from build123d import *

# Parameters (mm, degrees)
SKETCH2_W           = 94.999999992
SKETCH2_H           = 50.20499992
SKETCH2_R           = 1.5
SKETCH2_W_2         = 64.999999992
SKETCH2_H_2         = 20.20499992
BOSS_EXTRUDE2_DEPTH = 7


with BuildPart() as part:
    # Sketch2 → Boss-Extrude2 (new body)
    with BuildSketch(Plane(origin=(0, 0, 0), x_dir=(1, 0, 0), z_dir=(0, 1, 0))):
        Rectangle(SKETCH2_W, SKETCH2_H)
        with Locations(Location((-19.935762724, 17.60249996, 0), (0, 0, 270))):
            Circle(SKETCH2_R, mode=Mode.SUBTRACT)
        with Locations(Location((12.584576228, 17.60249996, 0), (0, 0, 270))):
            Circle(SKETCH2_R, mode=Mode.SUBTRACT)
        with Locations(Location((-39.970648897, 14.877942076, 0), (0, 0, 270))):
            Circle(SKETCH2_R, mode=Mode.SUBTRACT)
        with Locations(Location((-39.970648897, -2.517744737, 0), (0, 0, 270))):
            Circle(SKETCH2_R, mode=Mode.SUBTRACT)
        with Locations(Location((40.207477372, 12.990674167, 0), (0, 0, 270))):
            Circle(SKETCH2_R, mode=Mode.SUBTRACT)
        with Locations(Location((40.207477372, -3.666516508, 0), (0, 0, 270))):
            Circle(SKETCH2_R, mode=Mode.SUBTRACT)
        with Locations(Location((-13.716054438, -17.60249996, 0), (0, 0, 270))):
            Circle(SKETCH2_R, mode=Mode.SUBTRACT)
        with Locations(Location((6.580630125, -17.60249996, 0), (0, 0, 270))):
            Circle(SKETCH2_R, mode=Mode.SUBTRACT)
        Rectangle(SKETCH2_W_2, SKETCH2_H_2, mode=Mode.SUBTRACT)
    extrude(amount=BOSS_EXTRUDE2_DEPTH)


solid = part.part
Work out the finished part from the listing and answer in its coordinate system (mm). A direction names the side the tool comes from. Round coordinates to 2 decimals unless told otherwise and drop trailing zeros. Write each loop counter-clockwise with the first axis right and the second up, starting at its lowest first coordinate (ties: lowest second). Pieces come first, ordered by that corner, then holes. Notation, with made-up numbers: (49, 35) - (70, 35) arc R23 ccw to (70, 48) - close; hole circle Ø7 at (82.5, -33). An arc over 180 degrees is marked (long way). Answer in a Markdown table with one row per item. Add a question column.
1. A cutting plane is placed at A-A, the plane z = -8.5. Determine the outline of the cut face in (x, y).
2. The mould has two halves that part along Z. Classify faces 1 (the flat face through (0, 3, -10.102)), 2 (the flat face through (-1, 0, -12)), 3 (the flat face through (-1, 3, 25.102)), 4 (the cylindrical face through (6.647, 3.451, 16.104)): +Z half, -Z half, draft (parallel to the pull), parting line (faces both ways), or undercut.
3. A cutting plane is placed at B-B, the plane x = -5. Determine the outline of the cut face in (y, z), and give its area (3 significant figures).
4. For faces 5 (the flat face through (-1, 3, -25.102)), 6 (the flat face through (32.5, 3, 0)), determine the directions among +Z, -Z, +X, -X, +Y, -Y from which every point of the face is accessible in a straight line to the end or side of a thin tool.
5. Find the intervals of material crossed by line 1 along Z through (x, y) = (40, 6); line 2 along Z through (x, y) = (22.5, 4); line 3 along X through (y, z) = (2.25, -16.5), in increasing order. Write a range as from..to.
6. A cutting plane is placed at C-C, the plane y = 2. Count the separate pieces of the cut face and the enclosed holes in it, and give its area (3 significant figures).
Worked out:
| question | item | result |
|---|---|---|
| 1 | outline | (-47.5, 0) - (-32.5, 0) - (-32.5, 7) - (-47.5, 7) - close; (32.5, 0) - (47.5, 0) - (47.5, 7) - (32.5, 7) - close |
| 2 | face 1 | undercut |
| 2 | face 2 | draft |
| 2 | face 3 | +Z half |
| 2 | face 4 | undercut |
| 3 | outline | (0, -25.1) - (7, -25.1) - (7, -10.1) - (0, -10.1) - close; (0, 10.1) - (7, 10.1) - (7, 25.1) - (0, 25.1) - close |
| 3 | area | 210 mm^2 |
| 4 | face 5 | -Z, +X, -X, +Y, -Y |
| 4 | face 6 | +Y, -Y |
| 5 | line 1 | -25.1..-14.48, -11.51..2.18, 5.15..25.1 |
| 5 | line 2 | -25.1..-10.1, 10.1..25.1 |
| 5 | line 3 | -47.5..-20.95, -18.92..11.57, 13.6..47.5 |
| 6 | separate pieces | 1 |
| 6 | enclosed holes | 9 |
| 6 | area | 3,400 mm^2 |
